Input: part model. Units: mm. Frame: model coordinates. A direction names the side the tool comes from. Round coordinates to 2 decimals unless told otherwise and drop trailing zeros. Loops run counter-clockwise (first coordinate to the right, second up) from the corner with the lowest first, then second, coordinate; pieces in that order, holes last. Notation, with made-up numbers: (12, -23.5) -> (60, -23.5) arc R22 ccw to (60, -5.5) -> close; hole circle Ø10 at (37.5, -6.5). An arc over 180 degrees is marked (long way). Answer in a Markdown table with one row per item. Add a question column.
Q1. Pin query (flat end, axial travel): pin 1 (5 mm diameter, centred on x = -30, z = 15.5, fed in from +Y); pin 2 (10 mm diameter, centred on y = 63, z = 68, fed in from -X); pin 3 (1.4 mm diameter, centred on x = -162, z = 27.5, fed in from -Y); pin 4 (2 mm diameter, centred on y = 92.5, z = 28, fed in from +X). Return the tip coordinate at first contact, or that it passes through.
Q2. Section D-D, the plane x = -93.5. Output: boundary loops of the cut face in (y, z), and give its area (3 significant figures).
Q3. Ray query, L1, parallel to Y at x = -145, z = 73.5; L2, parallel to Y at x = -85.5, z = 67; L3, parallel to X at y = 98.5, z = 22.5. Return the intervals inside material, ascending. Write a range as from..to.
Q4. Mould query, pull axis Y, two halves, no side actions, for faces 1 (the face through (0.71, -5.01, 41.9)), 2 (the face through (0.73, -6.518, 41.905)), 3 (the face through (-39.144, 56.687, 9.887)). Classes: pulls with the +Y half, pulls with the -Y half, needs draft (parallel to the pull), parting line crosses it, or undercut.
Q5. Section A-A, the plane z = 15. Output: boundary loops of the cut face in (x, y), and give its area (3 significant figures).
Q6. Reachability of faces 4 (the face through (-162, 123.155, 42)), 5 (the face through (-162, 124.655, 42)), 6 (the face through (4.779, 15, 42)) from +Z, -Z, +X, -X, +Y, -Y: full face, straight path, thin tool, end or side. Return the list, or none.
Q7. Section B-B, the plane y = 24. Output: boundary loops of the cut face in (x, z), and give its area (4 significant figures).
Q8. Section C-C, the plane z = 49. Output: boundary loops of the cut face in (x, y), and give its area (3 significant figures).
```python
from build123d import *

# Parameters (mm, degrees)
BASE_FLANGE1_DEPTH = 85
SKETCH2_R          = 33.407017116
CUT_EXTRUDE1_DEPTH = 30


# Read off the part's stored shape, not the designer's step: Base-Flange1
with BuildPart() as part:
    # Base-Flange1 outline → Base-Flange1 (new body)
    with BuildSketch(Plane.XY):
        with BuildLine():
            ThreePointArc((4.779318239, -1.528186345), (4.767324577, -1.660569184), (4.731734161, -1.788640985))
            ThreePointArc((4.731734161, -1.788640985), (0.638889027, -5.018004141), (-4.132584418, -2.917240267))
            Line((-4.132584418, -2.917240267), (-5.358019189, -3.782289181))
            ThreePointArc((-5.358019189, -3.782289181), (0.828338715, -6.505992318), (6.134834735, -2.319026486))
            ThreePointArc((6.134834735, -2.319026486), (6.242900881, -1.930151397), (6.279318239, -1.528186345))
            Line((6.279318239, -1.528186345), (6.279318239, 30.807933335))
            ThreePointArc((6.279318239, 30.807933335), (5.972085307, 31.939269835), (5.134793267, 32.759791858))
            Line((5.134793267, 32.759791858), (-158.599410427, 124.369933097))
            ThreePointArc((-158.599410427, 124.369933097), (-159.127192628, 124.582318822), (-159.691485454, 124.654674574))
            Line((-159.691485454, 124.654674574), (-164.516949266, 124.654674574))
            Line((-164.516949266, 124.654674574), (-164.516949266, 123.154674574))
            Line((-164.516949266, 123.154674574), (-159.691485454, 123.154674574))
            ThreePointArc((-159.691485454, 123.154674574), (-159.50564172, 123.13084499), (-159.331822365, 123.060898051))
            Line((-159.331822365, 123.060898051), (4.402381329, 31.450756812))
            ThreePointArc((4.402381329, 31.450756812), (4.678134399, 31.180526765), (4.779318239, 30.807933335))
            Line((4.779318239, 30.807933335), (4.779318239, -1.528186345))
        make_face()
    extrude(amount=BASE_FLANGE1_DEPTH)

    # Sketch2 → Cut-Extrude1 (cut)
    with BuildSketch(Plane(origin=(15.183550365, 27.137459833, 0), x_dir=(0.872690030929894, -0.48827462550861755, 0), z_dir=(0.48827462550861755, 0.872690030929894, 0))):
        with Locations(Location((-69.081583233, -42.5, 0), (0, 0, 180))):
            Circle(SKETCH2_R)
    extrude(amount=-CUT_EXTRUDE1_DEPTH, mode=Mode.SUBTRACT)


solid = part.part
```
Answer block:
| question | item | result |
|---|---|---|
| 1 | pin 1 | y = 53 |
| 1 | pin 2 | through |
| 1 | pin 3 | y = 123.15 |
| 1 | pin 4 | x = -99.85 |
| 2 | outline | (86.23, 0) -> (87.95, 0) -> (87.95, 85) -> (86.23, 85) -> close |
| 2 | area | 146 mm^2 |
| 3 | L1 | 115.04..116.76 |
| 3 | L2 | 81.75..83.47 |
| 3 | L3 | -115.43..-112.36 |
| 4 | face 1 | undercut |
| 4 | face 2 | pulls with the -Y half |
| 4 | face 3 | parting line crosses it |
| 5 | outline | (-164.52, 123.15) -> (-159.69, 123.15) arc R0.74 cw to (-159.33, 123.06) -> (-62.39, 68.82) -> (-61.66, 70.13) -> (-158.6, 124.37) arc R2.24 ccw to (-159.69, 124.65) -> (-164.52, 124.65) -> close; (-29.28, 50.3) -> (4.4, 31.45) arc R0.74 cw to (4.78, 30.81) -> (4.78, -1.53) arc R0.74 cw to (4.73, -1.79) arc R5.06 cw to (-4.13, -2.92) -> (-5.36, -3.78) arc R6.56 ccw to (6.13, -2.32) arc R2.24 ccw to (6.28, -1.53) -> (6.28, 30.81) arc R2.24 ccw to (5.13, 32.76) -> (-28.55, 51.61) -> close |
| 5 | area | 303 mm^2 |
| 6 | face 4 | +Z, -Z, -X, -Y |
| 6 | face 5 | +Z, -Z, +X, -X, +Y |
| 6 | face 6 | +Z, -Z, -X |
| 7 | outline | (4.78, 0) -> (6.28, 0) -> (6.28, 85) -> (4.78, 85) -> close |
| 7 | area | 127.5 mm^2 |
| 8 | outline | (-164.52, 123.15) -> (-159.69, 123.15) arc R0.74 cw to (-159.33, 123.06) -> (-74.43, 75.56) -> (-73.7, 76.87) -> (-158.6, 124.37) arc R2.24 ccw to (-159.69, 124.65) -> (-164.52, 124.65) -> close; (-17.24, 43.56) -> (4.4, 31.45) arc R0.74 cw to (4.78, 30.81) -> (4.78, -1.53) arc R0.74 cw to (4.73, -1.79) arc R5.06 cw to (-4.13, -2.92) -> (-5.36, -3.78) arc R6.56 ccw to (6.13, -2.32) arc R2.24 ccw to (6.28, -1.53) -> (6.28, 30.81) arc R2.24 ccw to (5.13, 32.76) -> (-16.51, 44.87) -> close |
| 8 | area | 262 mm^2 |
